Design review of the part built by this model. Coordinates are the model's own, in mm. A direction names the side the tool comes from. Coordinates: 2 decimals unless noted, no trailing zeros. Write each loop counter-clockwise with the first axis right and the second up, starting at its lowest first coordinate (ties: lowest second). Pieces come first, ordered by that corner, then holes. Notation, with made-up numbers: (43, -27.75) - (100, -27.75) arc R18 ccw to (100, -2.75) - close; hole circle Ø6 at (9, -6.5). An arc over 180 degrees is marked (long way). One line per item, written item: value.
from build123d import *

# Parameters (mm, degrees)
SKETCH003_W      = 19.05
SKETCH003_H      = 5
EXTRUDE004_DEPTH = 17.78
SKETCH002_R      = 2.25
EXTRUDE003_DEPTH = 8
SKETCH001_R      = 1.05
EXTRUDE001_DEPTH = 10
SKETCH_W         = 6
SKETCH_H         = 6
EXTRUDE_DEPTH    = 14
BOX_W            = 70
BOX_H            = 30
BOX_DEPTH        = 5
SKETCH004_R      = 1.25
EXTRUDE006_DEPTH = 6
FILLET_R         = 1
FILLET001_R      = 1
FILLET002_R      = 1
FILLET003_R      = 1
FILLET004_R      = 1
FILLET005_R      = 1
FILLET006_R      = 1


with BuildPart() as extrude004:
    # Sketch003 (on Face2 of Fusion001) → Extrude004 (new body)
    with BuildSketch(Plane.XZ):
        with Locations((35, 2.5)):
            Rectangle(SKETCH003_W, SKETCH003_H)
    extrude(amount=EXTRUDE004_DEPTH)


with BuildPart() as extrude003:
    # Sketch002 (on Face7 of Fusion) → Extrude003 (new body)
    with BuildSketch(Plane(origin=(0, 0, 0), x_dir=(1, 0, 0), z_dir=(0, 0, -1))):
        with Locations((42.5, -7)):
            Circle(SKETCH002_R)
        with Locations((27.5, -7)):
            Circle(SKETCH002_R)
        with Locations((57.5, -7)):
            Circle(SKETCH002_R)
        with Locations((12.5, -7)):
            Circle(SKETCH002_R)
        with Locations((42.5, -22)):
            Circle(SKETCH002_R)
        with Locations((57.5, -22)):
            Circle(SKETCH002_R)
        with Locations((12.5, -22)):
            Circle(SKETCH002_R)
        with Locations((27.5, -22)):
            Circle(SKETCH002_R)
    extrude(amount=EXTRUDE003_DEPTH)


with BuildPart() as extrude001:
    # Sketch001 (on Face24 of Extrude) → Extrude001 (new body)
    with BuildSketch(Plane.XY.offset(19)):
        with Locations((3, 27)):
            Circle(SKETCH001_R)
        with Locations((3, 3)):
            Circle(SKETCH001_R)
        with Locations((67, 3)):
            Circle(SKETCH001_R)
        with Locations((67, 27)):
            Circle(SKETCH001_R)
    extrude(amount=-EXTRUDE001_DEPTH)


with BuildPart() as cut:
    # Sketch (on Face6 of Box) → Extrude (new body)
    with BuildSketch(Plane.XY.offset(5)):
        with Locations((3, 27)):
            Rectangle(SKETCH_W, SKETCH_H)
        with Locations((3, 3)):
            Rectangle(SKETCH_W, SKETCH_H)
        with Locations((67, 3)):
            Rectangle(SKETCH_W, SKETCH_H)
        with Locations((67, 27)):
            Rectangle(SKETCH_W, SKETCH_H)
    extrude(amount=EXTRUDE_DEPTH)

    # Cut: cut Extrude001
    add(extrude001.part, mode=Mode.SUBTRACT)


with BuildPart() as fusion001:
    # Box → Box (new body)
    with BuildSketch(Plane.XY):
        with Locations((35, 15)):
            Rectangle(BOX_W, BOX_H)
    extrude(amount=BOX_DEPTH)

    # Fusion: union Cut
    add(cut.part)

    # Fusion001: union Extrude003
    add(extrude003.part)


with BuildPart() as speaker_plate:
    # Sketch004 (on Face4 of Extrude004) → Extrude006 (new body)
    with BuildSketch(Plane.XY.offset(5)):
        with Locations((28.015, -2.54)):
            Circle(SKETCH004_R)
        with Locations((28.015, -15.24)):
            Circle(SKETCH004_R)
    extrude(amount=EXTRUDE006_DEPTH)

    # Fusion002: union Extrude004, Fusion001
    add(extrude004.part)
    add(fusion001.part)

    # Fillet
    fillet_edges = [speaker_plate.edges().sort_by_distance(p)[0] for p in [
        (0, 0, 2.5),
        (0, 0, 12),
    ]]
    fillet(fillet_edges, radius=FILLET_R)

    # Fillet001
    fillet001_edges = [speaker_plate.edges().sort_by_distance(p)[0] for p in [
        (25.475, 0, 2.5),
        (25.475, -17.78, 2.5),
    ]]
    fillet(fillet001_edges, radius=FILLET001_R)

    # Fillet002
    fillet002_edges = [speaker_plate.edges().sort_by_distance(p)[0] for p in [
        (44.525, -17.78, 2.5),
    ]]
    fillet(fillet002_edges, radius=FILLET002_R)

    # Fillet003
    fillet003_edges = [speaker_plate.edges().sort_by_distance(p)[0] for p in [
        (44.525, 0, 2.5),
    ]]
    fillet(fillet003_edges, radius=FILLET003_R)

    # Fillet004
    fillet004_edges = [speaker_plate.edges().sort_by_distance(p)[0] for p in [
        (70, 0, 2.5),
        (70, 0, 12),
    ]]
    fillet(fillet004_edges, radius=FILLET004_R)

    # Fillet005
    fillet005_edges = [speaker_plate.edges().sort_by_distance(p)[0] for p in [
        (70, 30, 2.5),
        (70, 30, 12),
    ]]
    fillet(fillet005_edges, radius=FILLET005_R)

    # Fillet006
    fillet006_edges = [speaker_plate.edges().sort_by_distance(p)[0] for p in [
        (0, 30, 2.5),
        (0, 30, 12),
    ]]
    fillet(fillet006_edges, radius=FILLET006_R)


solid = speaker_plate.part
1. Wall thickness on line 1 along Y through (x, z) = (3, 14.75); line 2 along Y through (x, z) = (5.5, 9); line 3 along X through (y, z) = (-3, 3) (3 decimals): over which ranges is each line inside the solid? List them lowest first.
Answer block:
line 1: y = 0 to 1.95, 4.05 to 6, 24 to 25.95, 28.05 to 30
line 2: y = 0 to 6, 24 to 30
line 3: x = 25.475 to 44.525
2. For faces 4 (the face through (12.012, 24.196, -3.944)), 5 (the face through (57, 7, -8)), 6 (the face through (35, 12, 5)), 7 (the face through (3, 24, 12)), list the 3-axis set-ups (+Z, -Z, +X, -X, +Y, -Y) from which the entire face can be reached by the end or side of a thin tool; tool diameter is ignored.
Answer block:
face 4: -Z
face 5: -Z, +X, -X, +Y, -Y
face 6: +Z
face 7: +Z, +X, -X
3. Insertion check: pin 1 Ø2.5 at (y, z) = (-11.5, 3.5) entering from +X (3 decimals); pin 2 Ø1.8 at (x, z) = (4, 11) entering from -Y; pin 3 Ø4 at (x, y) = (37.5, -6.5) entering from +Z; pin 4 Ø12 at (y, z) = (17.5, -1.5) entering from +X. Each pin has a flat end and moves straight along its axis. Give the tip position at first contact, or say it passes through.
Answer block:
pin 1: stops at x = 44.525
pin 2: stops at y = 0
pin 3: stops at z = 5
pin 4: stops at x = 70
4. Consider section D-D, the plane y = -2.54. Write out the cut boundary in (x, z) (3 decimals), then the cut area to 3 significant figures.
Answer block:
outline: (25.475, 0) - (44.525, 0) - (44.525, 5) - (29.265, 5) - (29.265, 11) - (26.765, 11) - (26.765, 5) - (25.475, 5) - close
area: 110 mm^2
5. Consider section C-C, the plane x = 12.5. Write out the cut boundary in (y, z).
Answer block:
outline: (0, 0) - (4.75, 0) - (4.75, -8) - (9.25, -8) - (9.25, 0) - (19.75, 0) - (19.75, -8) - (24.25, -8) - (24.25, 0) - (30, 0) - (30, 5) - (0, 5) - close
6. Consider section B-B, the plane z = -3.5. Write out the cut boundary in (x, y), then the cut area to 3 significant figures.
Answer block:
outline: circle Ø4.5 at (12.5, 7); circle Ø4.5 at (12.5, 22); circle Ø4.5 at (27.5, 7); circle Ø4.5 at (27.5, 22); circle Ø4.5 at (42.5, 7); circle Ø4.5 at (42.5, 22); circle Ø4.5 at (57.5, 7); circle Ø4.5 at (57.5, 22)
area: 127 mm^2
7. Mouldability with a two-part tool opening along Y and no side actions: class faces 1 (the face through (55.252, 6.901, -3.944)), 2 (the face through (70, 15, 3)), 3 (the face through (62, 0, 3)) as released by +Y, released by -Y, zero draft, split by the parting line, or undercut.
Answer block:
face 1: undercut
face 2: zero draft
face 3: released by -Y
8. Consider section A-A, the plane z = 15.25. Write out the cut boundary in (x, y), then the cut area to 3 significant figures.
Answer block:
outline: (0, 1) arc R1 ccw to (1, 0) - (6, 0) - (6, 6) - (0, 6) - close; (0, 24) - (6, 24) - (6, 30) - (1, 30) arc R1 ccw to (0, 29) - close; (64, 0) - (69, 0) arc R1 ccw to (70, 1) - (70, 6) - (64, 6) - close; (64, 24) - (70, 24) - (70, 29) arc R1 ccw to (69, 30) - (64, 30) - close; hole circle Ø2.1 at (3, 3); hole circle Ø2.1 at (3, 27); hole circle Ø2.1 at (67, 3); hole circle Ø2.1 at (67, 27)
area: 129 mm^2
